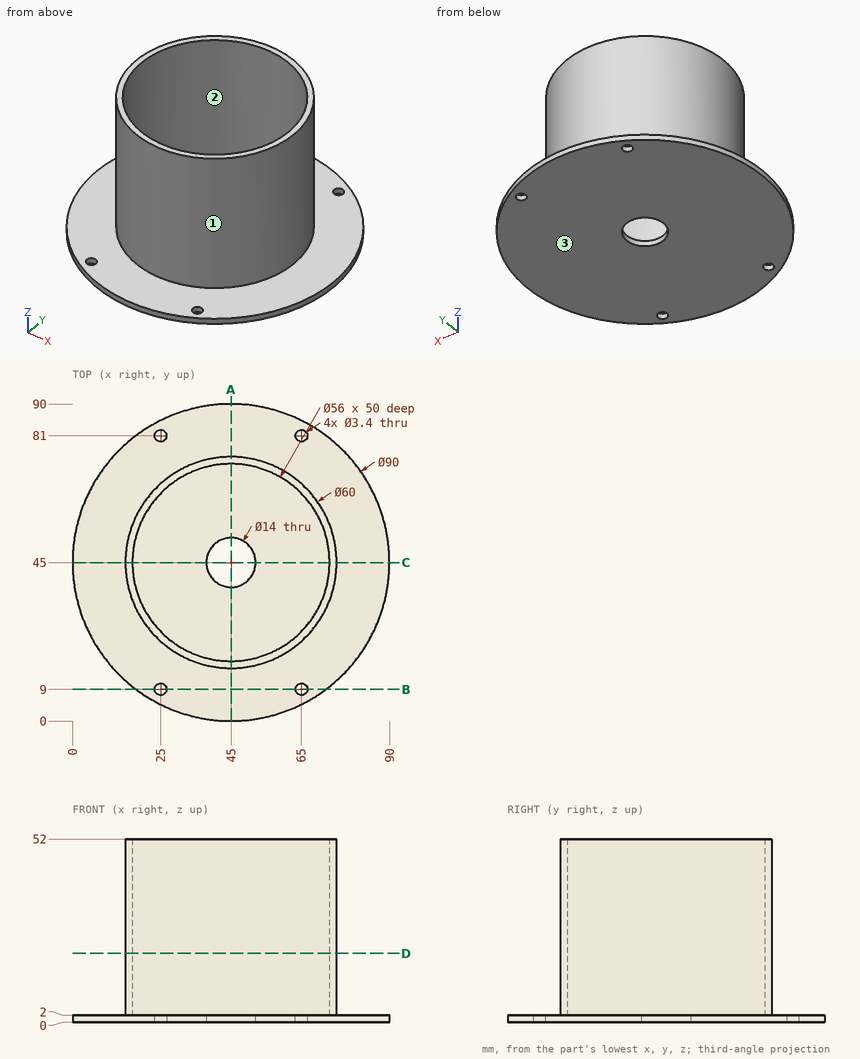
Check sheet for the drawn part. Datum: minimum x, y, z corner. Units: mm. Coordinates: 2 decimals unless noted, no trailing zeros. Loops run counter-clockwise (first coordinate to the right, second up) from the corner with the lowest first, then second, coordinate; pieces in that order, holes last. Notation, with made-up numbers: (73, 48.5) - (77, 48.5) arc R8 ccw to (77, 53.5) - close; hole circle Ø2 at (18.5, 68.25). An arc over 180 degrees is marked (long way). Put each result on its own line as item: value.
Item 1: Scan lines: line 1 along Y through (x, z) = (45, 34); line 2 along Y through (x, z) = (45, 1.55); line 3 along Z through (x, y) = (58.5, 49.5). Record each from-to range of solid material in increasing order.
Conclusion:
line 1: y = 15 to 17, 73 to 75
line 2: y = 0 to 38, 52 to 90
line 3: z = 0 to 2
Item 2: Section check B-B (y = 9). Enter the section's corners in (x, z), then the cut area to 3 significant figures.
Conclusion:
outline: (18, 0) - (23.3, 0) - (23.3, 2) - (18, 2) - close; (26.7, 0) - (63.3, 0) - (63.3, 2) - (26.7, 2) - close; (66.7, 0) - (72, 0) - (72, 2) - (66.7, 2) - close
area: 94.4 mm2
Item 3: Section check A-A (x = 45). Enter the section's corners in (y, z).
Conclusion:
outline: (0, 0) - (38, 0) - (38, 2) - (17, 2) - (17, 52) - (15, 52) - (15, 2) - (0, 2) - close; (52, 0) - (90, 0) - (90, 2) - (75, 2) - (75, 52) - (73, 52) - (73, 2) - (52, 2) - close
Item 4: Gauge pin test, flat ends, axial feed: pin 1 Ø6 at (y, z) = (41, 8.5) entering from -X; pin 2 Ø8 at (y, z) = (26.5, 10.5) entering from -X; pin 3 Ø10 at (y, z) = (46.5, 27) entering from +X. Record the tip position at first contact, or that the pin passes through.
Conclusion:
pin 1: stops at x = 15.02
pin 2: stops at x = 18.74
pin 3: stops at x = 75
Item 5: Draft check along Y on the marked faces 1, 2 and 3. Enter one of: pulls with the +Y half, pulls with the -Y half, needs draft (parallel to the pull), parting line crosses it, or undercut.
Conclusion:
face 1: parting line crosses it
face 2: undercut
face 3: needs draft
Item 6: Section check D-D (z = 19.5). Enter the section's corners in (x, y), then the cut area to 3 significant figures.
Conclusion:
outline: circle Ø60 at (45, 45); hole circle Ø56 at (45, 45)
area: 364 mm2
